Source: CAD feature listing. Evaluate the final solid. Frame: model axes, mm. A direction names the side the tool comes from. Give positions to 0.01 mm unless a question says otherwise; leave off trailing zeros. Order: outer loops, then holes, each group sorted by start corner. A loop starts at its lowest first (then second) coordinate and runs counter-clockwise, first axis right, second up.
1) Material intervals for line 1 (Z direction, x = -25, y = 10.8); line 2 (X direction, y = 5.5, z = -21); line 3 (Z direction, x = 0, y = 11.95), sorted ascending.
2) Section A-A, the plane x = 0. Return loops of the section in (y, z), plus the area to 3 significant figures.
3) First-contact query: P1, Ø1, axis at x = -19, z = 14.5, coming from the -Y side; P2, Ø6, axis at x = -37.5, z = -25.5, coming from the +Y side; P3, Ø3.5, axis at x = -40, z = 16, coming from the +Y side. Flat tips, straight axial feed; report the tip coordinate or a pass-through.
4) Draft query along Z for faces 4 (the face through (48, 6, 34)), 5 (the face through (-39.9, 3.4, 11.8)). Return one class per face: released by +Z, released by -Z, zero draft, split by the parting line, or undercut.
5) Section B-B, the plane y = 2.75. Give the number of separate pieces and of enclosed holes in the cut face, plus the area to 3 significant figures.
6) Access query for faces 1 (the face through (-39.866, 12.335, -8.916)), 2 (the face through (40.073, 0.365, 11.665)), 3 (the face through (40.1, 3.4, 28.2)). Directions: +Z, -Z, +X, -X, +Y, -Y. A direction counts if a zero-diameter tool reaches every point of the face in a straight line with its end or side. Return the directions, or none.
```python
from build123d import *

# Parameters (mm, degrees)
SKETCH1_W           = 100
SKETCH1_H           = 70
BOSS_EXTRUDE1_DEPTH = 12.7
SKETCH2_R           = 25
CUT_EXTRUDE1_DEPTH  = 3
SKETCH3_R           = 10
CUT_EXTRUDE2_DEPTH  = 10.7
SKETCH4_R           = 2.1
CUT_EXTRUDE3_DEPTH  = 13.7
SKETCH5_W           = 60.5
SKETCH5_H           = 60.5
CUT_EXTRUDE4_DEPTH  = 7
FILLET1_R           = 3
FILLET2_R           = 5
CUT_EXTRUDE5_DEPTH  = 13.7
SKETCH7_R           = 25.25
CUT_EXTRUDE6_DEPTH  = 3.2
CUT_EXTRUDE7_DEPTH  = 6
CHAMFER1_SIZE       = 0.5


with BuildPart() as part:
    # Sketch1 → Boss-Extrude1 (new body)
    with BuildSketch(Plane(origin=(0, 0, 0), x_dir=(1, 0, 0), z_dir=(0, 1, 0))):
        Rectangle(SKETCH1_W, SKETCH1_H)
    extrude(amount=BOSS_EXTRUDE1_DEPTH)

    # Sketch2 → Cut-Extrude1 (cut)
    with BuildSketch(Plane.XZ):
        Circle(SKETCH2_R)
    extrude(amount=-CUT_EXTRUDE1_DEPTH, mode=Mode.SUBTRACT)

    # Sketch3 → Cut-Extrude2 (cut, through all)
    with BuildSketch(Plane.XZ.offset(-3)):
        Circle(SKETCH3_R)
    extrude(amount=-CUT_EXTRUDE2_DEPTH, mode=Mode.SUBTRACT)

    # Sketch4 → Cut-Extrude3 (cut, through all)
    with BuildSketch(Plane.XZ):
        with Locations((-25, 25)):
            Circle(SKETCH4_R)
        with Locations((25, 25)):
            Circle(SKETCH4_R)
        with Locations((25, -25)):
            Circle(SKETCH4_R)
        with Locations((-25, -25)):
            Circle(SKETCH4_R)
    extrude(amount=-CUT_EXTRUDE3_DEPTH, mode=Mode.SUBTRACT)

    # Sketch5 → Cut-Extrude4 (cut)
    with BuildSketch(Plane.XZ):
        Rectangle(SKETCH5_W, SKETCH5_H)
    extrude(amount=-CUT_EXTRUDE4_DEPTH, mode=Mode.SUBTRACT)

    # Fillet1
    fillet1_edges = [part.edges().sort_by_distance(p)[0] for p in [
        (-30.25, 3.5, -30.25),
        (-30.25, 3.5, 30.25),
        (30.25, 3.5, 30.25),
        (30.25, 3.5, -30.25),
    ]]
    fillet(fillet1_edges, radius=FILLET1_R)

    # Fillet2
    fillet2_edges = [part.edges().sort_by_distance(p)[0] for p in [
        (-50, 6.35, -35),
        (50, 6.35, -35),
        (50, 6.35, 35),
        (-50, 6.35, 35),
    ]]
    fillet(fillet2_edges, radius=FILLET2_R)

    # Sketch6 → Cut-Extrude5 (cut, through all)
    with BuildSketch(Plane(origin=(0, 12.7, 0), x_dir=(1, 0, 0), z_dir=(0, 1, 0))):
        with BuildLine():
            Line((-36.8, 25), (-36.8, 15))
            ThreePointArc((-36.8, 15), (-40, 11.8), (-43.2, 15))
            Line((-43.2, 15), (-43.2, 25))
            ThreePointArc((-43.2, 25), (-40, 28.2), (-36.8, 25))
        make_face()
        with BuildLine():
            Line((-36.8, -25), (-36.8, -15))
            ThreePointArc((-36.8, -15), (-40, -11.8), (-43.2, -15))
            Line((-43.2, -15), (-43.2, -25))
            ThreePointArc((-43.2, -25), (-40, -28.2), (-36.8, -25))
        make_face()
        with BuildLine():
            Line((36.8, -25), (36.8, -15))
            ThreePointArc((36.8, -15), (40, -11.8), (43.2, -15))
            Line((43.2, -15), (43.2, -25))
            ThreePointArc((43.2, -25), (40, -28.2), (36.8, -25))
        make_face()
        with BuildLine():
            Line((36.8, 25), (36.8, 15))
            ThreePointArc((36.8, 15), (40, 11.8), (43.2, 15))
            Line((43.2, 15), (43.2, 25))
            ThreePointArc((43.2, 25), (40, 28.2), (36.8, 25))
        make_face()
    extrude(amount=-CUT_EXTRUDE5_DEPTH, mode=Mode.SUBTRACT)

    # Sketch7 → Cut-Extrude6 (cut)
    with BuildSketch(Plane.XZ.offset(-7)):
        Circle(SKETCH7_R)
    extrude(amount=-CUT_EXTRUDE6_DEPTH, mode=Mode.SUBTRACT)

    # Sketch9 → Cut-Extrude7 (cut)
    with BuildSketch(Plane(origin=(0, 12.7, 0), x_dir=(1, 0, 0), z_dir=(0, 1, 0))):
        with BuildLine():
            Line((45.95, 15), (45.95, 25))
            ThreePointArc((45.95, 25), (40, 30.95), (34.05, 25))
            Line((34.05, 25), (34.05, 15))
            ThreePointArc((34.05, 15), (40, 9.05), (45.95, 15))
        make_face()
        with BuildLine():
            Line((34.05, -25), (34.05, -15))
            ThreePointArc((34.05, -15), (40, -9.05), (45.95, -15))
            Line((45.95, -15), (45.95, -25))
            ThreePointArc((45.95, -25), (40, -30.95), (34.05, -25))
        make_face()
        with BuildLine():
            Line((-45.95, -15), (-45.95, -25))
            ThreePointArc((-45.95, -25), (-40, -30.95), (-34.05, -25))
            Line((-34.05, -25), (-34.05, -15))
            ThreePointArc((-34.05, -15), (-40, -9.05), (-45.95, -15))
        make_face()
        with BuildLine():
            Line((-34.05, 25), (-34.05, 15))
            ThreePointArc((-34.05, 15), (-40, 9.05), (-45.95, 15))
            Line((-45.95, 15), (-45.95, 25))
            ThreePointArc((-45.95, 25), (-40, 30.95), (-34.05, 25))
        make_face()
    extrude(amount=-CUT_EXTRUDE7_DEPTH, mode=Mode.SUBTRACT)

    # Chamfer1
    chamfer1_edges = [part.edges().sort_by_distance(p)[0] for p in [
        (40, 0, -28.2),
        (43.2, 0, -20),
        (40, 0, -11.8),
        (36.8, 0, -20),
        (40, 0, 28.2),
        (36.8, 0, 20),
        (40, 0, 11.8),
        (43.2, 0, 20),
        (-40, 0, 28.2),
        (-43.2, 0, 20),
        (-40, 0, 11.8),
        (-36.8, 0, 20),
        (-40, 0, -28.2),
        (-36.8, 0, -20),
        (-40, 0, -11.8),
        (-43.2, 0, -20),
        (-25.25, 7, 0),
        (-10, 10.2, 0),
        (36.8, 6.7, -20),
        (43.2, 6.7, 20),
        (-36.8, 6.7, 20),
        (-43.2, 6.7, -20),
        (-10, 12.7, 0),
        (40, 12.7, -9.05),
        (45.95, 12.7, -20),
        (40, 12.7, -30.95),
        (34.05, 12.7, -20),
        (40, 6.7, -28.2),
        (43.2, 6.7, -20),
        (40, 6.7, -11.8),
        (-36.8, 6.7, -20),
        (-40, 6.7, -28.2),
        (-40, 6.7, -11.8),
        (-40, 12.7, -30.95),
        (-45.95, 12.7, -20),
        (-40, 12.7, -9.05),
        (-34.05, 12.7, -20),
        (-40, 12.7, 9.05),
        (-45.95, 12.7, 20),
        (-40, 12.7, 30.95),
        (-34.05, 12.7, 20),
        (-40, 6.7, 28.2),
        (-43.2, 6.7, 20),
        (-40, 6.7, 11.8),
        (36.8, 6.7, 20),
        (40, 6.7, 28.2),
        (40, 6.7, 11.8),
        (40, 12.7, 30.95),
        (45.95, 12.7, 20),
        (40, 12.7, 9.05),
        (34.05, 12.7, 20),
        (-27.1, 12.7, -25),
        (22.9, 12.7, -25),
        (22.9, 12.7, 25),
        (-27.1, 12.7, 25),
        (-27.1, 7, 25),
        (22.9, 7, 25),
        (22.9, 7, -25),
        (-27.1, 7, -25),
        (-50, 0, 0),
        (-50, 12.7, 0),
        (0, 0, -35),
        (50, 0, 0),
        (0, 0, 35),
        (48.535533906, 0, 33.535533906),
        (-48.535533906, 0, 33.535533906),
        (48.535533906, 0, -33.535533906),
        (-48.535533906, 0, -33.535533906),
        (0, 12.7, -35),
        (0, 12.7, 35),
        (50, 12.7, 0),
        (48.535533906, 12.7, 33.535533906),
        (-48.535533906, 12.7, 33.535533906),
        (48.535533906, 12.7, -33.535533906),
        (-48.535533906, 12.7, -33.535533906),
    ]]
    chamfer(chamfer1_edges, length=CHAMFER1_SIZE)


solid = part.part
```
From the geometry:
1. line 1: z = -35 to -27.1, -22.9 to 22.9, 27.1 to 35
1. line 2: x = -50 to -43.2, -36.8 to -30.25, 30.25 to 36.8, 43.2 to 50
1. line 3: z = -35 to -10, 10 to 35
2. outline: (0, -34.5) - (0.5, -35) - (12.2, -35) - (12.7, -34.5) - (12.7, -10.5) - (12.2, -10) - (10.7, -10) - (10.2, -10.5) - (10.2, -25.25) - (7.5, -25.25) - (7, -25.75) - (7, -30.25) - (0, -30.25) - close; (0, 30.25) - (7, 30.25) - (7, 25.75) - (7.5, 25.25) - (10.2, 25.25) - (10.2, 10.5) - (10.7, 10) - (12.2, 10) - (12.7, 10.5) - (12.7, 34.5) - (12.2, 35) - (0.5, 35) - (0, 34.5) - close
2. area: 253 mm2
3. P1: stops at y = 10.2
3. P2: stops at y = 6.7
3. P3: passes through
4. face 4: released by +Z
4. face 5: undercut
5. separate pieces: 1
5. enclosed holes: 5
5. area: 2,940 mm2
6. face 1: +Y
6. face 2: -Y
6. face 3: +Y, -Y
